```python
from build123d import *

# Parameters (mm, degrees)
F0_R     = 15.9004
F1_DEPTH = 7.239
F2_R     = 1.89865
F3_DEPTH = 14.479
F6_W     = 3.175
F6_H     = 7.62
F6_W_2   = 7.62
F6_H_2   = 3.175


with BuildPart() as f1:
    # F0 (on Top) → F1 (new body, symmetric)
    with BuildSketch(Plane.XY):
        Circle(F0_R)
    extrude(amount=F1_DEPTH, both=True)

    # F2 (on face) → F3 (cut, through all)
    with BuildSketch(Plane.XY.offset(7.239)):
        Circle(F2_R)
    extrude(amount=-F3_DEPTH, mode=Mode.SUBTRACT)

    # F4 (on Right) → F5 (revolve, cut)
    with BuildSketch(Plane.YZ):
        Polygon((7.62, 0), (12.3317, -4.7117), (16.1773537484, -4.7117), (16.1773537484, 4.7117), (12.3317, 4.7117), align=None)
        Polygon((11.7093047491, 8.5794328097), (5.715, 8.5794328097), (5.715, 2.5851280605), align=None)
    revolve(axis=Axis((0, 0, 6.2945708632), (0, 0, 1)), mode=Mode.SUBTRACT)

    # F6 (on face) → F7 (join, up to the next surface of F1)
    with BuildSketch(Plane.XY.offset(7.239)):
        with Locations((0, 8.4708621725)):
            Rectangle(F6_W, F6_H)
        with Locations((-8.4708621725, 0)):
            Rectangle(F6_W_2, F6_H_2)
        with Locations((0, -8.4708621725)):
            Rectangle(F6_W, F6_H)
        with Locations((8.4708621725, 0)):
            Rectangle(F6_W_2, F6_H_2)
    extrude(until=Until.NEXT, dir=(0, 0, -1))


solid = f1.part
```
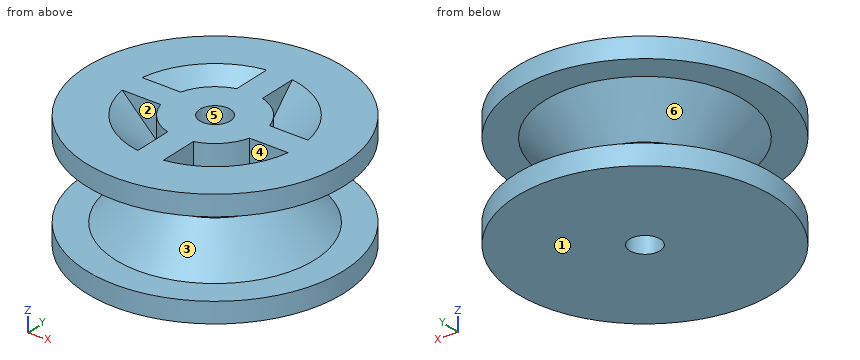
Source: CAD feature listing. Evaluate the final solid. Frame: model axes, mm. Face numbers are marked on the shaded views. A direction names the side the tool comes from. Round coordinates to 2 decimals unless told otherwise and drop trailing zeros. Loops run counter-clockwise (first coordinate to the right, second up) from the corner with the lowest first, then second, coordinate; pieces in that order, holes last.
1. Contact query for flat-ended pins moving along their axis: pin 1 (5 mm diameter, centred on y = -9, z = 4, fed in from -X); pin 2 (5 mm diameter, centred on x = -9, z = 5.5, fed in from +Y); pin 3 (3.5 mm diameter, centred on y = 7, z = 4, fed in from +X); pin 4 (3 mm diameter, centred on x = 0, y = 0, fed in from +Z). Output: stop coordinate, or through.
2. Ray query, L1, parallel to Z at x = 14, y = -1.5; L2, parallel to X at y = -4, z = 5.75; L3, parallel to Z at x = -6, y = 10.5. Return the intervals inside material, ascending.
3. Section query C-C on z = 1.5. Output: boundary loops of the cut face in (x, y), and give its area (3 significant figures).
4. Section query A-A on z = -3.5. Output: boundary loops of the cut face in (x, y).
5. Section query B-B on z = 3.25. Output: boundary loops of the cut face in (x, y) (1 decimal), and give its area (3 significant figures).
6. Mould query, pull axis Z, two halves, no side actions, for the marked faces 1, 2 and 3. Classes: released by +Z, released by -Z, zero draft, split by the parting line, or undercut.
7. Access query for the marked faces 4, 5 and 6. Directions: +Z, -Z, +X, -X, +Y, -Y. A direction counts if a zero-diameter tool reaches every point of the face in a straight line with its end or side. Return the directions, or none.
Answers below:
1. pin 1: stops at x = -14.46
1. pin 2: stops at y = 14.51
1. pin 3: stops at x = 14.95
1. pin 4: passes through
2. L1: z = -7.24 to -4.71, 4.71 to 7.24
2. L2: x = -15.39 to -7.93, -4.08 to 4.08, 7.93 to 15.39
2. L3: z = -7.24 to -4.47, 4.47 to 7.24
3. outline: circle Ø18.24 at (0, 0); hole circle Ø3.8 at (0, 0)
3. area: 250 mm2
4. outline: circle Ø22.24 at (0, 0); hole circle Ø3.8 at (0, 0)
5. outline: circle Ø21.7 at (0, 0); hole (-6.2, -1.6) arc R6.4 ccw to (-1.6, -6.2) - (-1.6, -5.5) arc R5.7 cw to (-5.5, -1.6) - close; hole (-6.2, 1.6) - (-5.5, 1.6) arc R5.7 cw to (-1.6, 5.5) - (-1.6, 6.2) arc R6.4 ccw to start; hole circle Ø3.8 at (0, 0); hole (1.6, -6.2) arc R6.4 ccw to (6.2, -1.6) - (5.5, -1.6) arc R5.7 cw to (1.6, -5.5) - close; hole (1.6, 5.5) arc R5.7 cw to (5.5, 1.6) - (6.2, 1.6) arc R6.4 ccw to (1.6, 6.2) - close
5. area: 343 mm2
6. face 1: released by -Z
6. face 2: zero draft
6. face 3: undercut
7. face 4: +Z
7. face 5: +Z, -Z
7. face 6: none
